The listing builds one solid part. Answer for the finished solid, in the listing's coordinates (mm). A direction names the side the tool comes from. Give positions to 0.01 mm unless a question says otherwise; leave off trailing zeros. Loops run counter-clockwise (first coordinate to the right, second up) from the corner with the lowest first, then second, coordinate; pieces in that order, holes last.
Item 1: A tool of negligible diameter and unlimited length cuts with its end or side. For faces 1 (the face through (5.7, 17, 0)), 2 (the face through (0, 1.1, 2.7)), from which of +Z, -Z, +X, -X, +Y, -Y can it reach the whole face along a straight path? Write none if from no direction.
Item 2: Consider line 1 along Z through (x, y) = (0, 1.5); line 2 along Y through (x, z) = (4, -4.5); line 3 along Y through (x, z) = (1.25, -2). Determine where each line is inside the solid, lowest interval first.
Item 3: Section C-C, the plane y = 11.25 is taken. Give the vertices of the cut face in (x, z).
Item 4: Section D-D, the plane z = 4.5 is taken. Give the vertices of the cut face in (x, y).
Item 5: The mould has two halves that part along Z. Classify faces 3 (the face through (-5.15, 11.5, -0.08)), 4 (the face through (0, 5, -1.7)), 5 (the face through (0, 17, -5.7)): pulls with the +Z half, pulls with the -Z half, needs draft (parallel to the pull), parting line crosses it, or undercut.
Item 6: Each of these flat-tipped pins is pushed along its axis until it touches: pin 1 Ø5 at (x, y) = (0.5, 4.5) entering from -Z; pin 2 Ø1.1 at (y, z) = (4, 0.5) entering from +X; pin 3 Ø1.1 at (y, z) = (2.5, 0.5) entering from -X. Where does it stop, or does it pass through?
Item 7: Section A-A, the plane y = 7.75 is taken. Give the vertices of the cut face in (x, z) (1 decimal).
Item 8: Section B-B, the plane x = 0 is taken. Give the vertices of the cut face in (y, z), and give its area (3 significant figures).
Autodesk Inventor part; units mm, degrees
ref_plane "YZ Plane" through (0, 0, 0) normal (1, 0, 0) x (0, 1, 0)
ref_plane "XZ Plane" through (0, 0, 0) normal (0, 1, 0) x (-1, 0, 0)
ref_plane "XY Plane" through (0, 0, 0) normal (0, 0, 1) x (1, 0, 0)
sketch "Sketch1" plane through (0, 0, 0) normal (0, 1, 0) x (-1, 0, 0)
  line L0 (14.5, -14.5) -> (-14.5, -14.5)
  line L1 (-14.5, -14.5) -> (-14.5, 14.5)
  line L2 (-14.5, 14.5) -> (14.5, 14.5)
  line L3 (14.5, 14.5) -> (14.5, -14.5)
  circle A0 centre (0, 0) radius 4
  dimension "d11" = 29
  dimension "d14" = 29
  dimension "d31" = 8
extrude "Extrusion1" add sketch "Sketch1" along normal blind 11.5 contours A0
sketch "Sketch2" plane through (0, 11.5, 0) normal (0, 1, 0) x (1, 0, 0)
  line L0 (-5.7, 5.7) -> (5.7, 5.7)
  line L1 (5.7, 5.7) -> (5.7, -5.7)
  line L2 (5.7, -5.7) -> (-5.7, -5.7)
  line L3 (-5.7, -5.7) -> (-5.7, 5.7)
  line L4 (14.5, 14.5) -> (-14.5, 14.5)
  line L5 (14.5, -14.5) -> (14.5, 14.5)
  line L6 (-14.5, -14.5) -> (14.5, -14.5)
  line L7 (-14.5, 14.5) -> (-14.5, -14.5)
  point P0 (0, 0)
  dimension "d15" = 8.8
  dimension "d16" = 8.8
  dimension "d17" = 8.8
  dimension "d18" = 8.8
  dimension "d32" = 11.4
extrude "Extrusion2" add sketch "Sketch2" along normal blind 11 contours L0 L1 L2 L3
sketch "Sketch3" plane through (0, 0, 0) normal (0, -1, 0) x (1, 0, 0)
  line L0 (-0.0005, -0.0003) -> (-0.0005, -1.7003)
  line L1 (-0.0005, -1.7003) -> (2.6995, -1.7003)
  line L2 (2.6995, -1.7003) -> (2.6995, 1.6997)
  line L3 (2.6995, 1.6997) -> (-2.7005, 1.6997)
  line L4 (-2.7005, 1.6997) -> (-2.7005, -1.7003)
  line L5 (-2.7005, -1.7003) -> (-0.0005, -1.7003)
  dimension "d42" = 1.7
  dimension "d43" = 2.7
  dimension "d44" = 3.4
  dimension "d45" = 5.4
extrude "Extrusion3" cut sketch "Sketch3" against normal blind 8.2
sketch "Sketch5" plane through (0, 0, 0) normal (0, -1, 0) x (1, 0, 0)
  circle A0 centre (0, 0) radius 2.7
  dimension "d35" = 5.4
extrude "Extrusion4" cut sketch "Sketch5" against normal blind 2.2
fillet "Fillet1" radius 0.635 4 edges at (2.6995, 4.1, 1.6997) (2.6995, 4.1, -1.7003) (-2.7005, 4.1, -1.7003) (-2.7005, 4.1, 1.6997)
sketch "Sketch6" plane through (0, 11.5, 0) normal (0, -1, 0) x (1, 0, 0)
  circle A0 centre (0, 0) radius 5
  dimension "d47" = 10
extrude "Extrusion5" add sketch "Sketch6" along normal up to surface (3.3 mm away)
equation "\"d14\" = d11"
equation "\"d16\" = d15"
equation "\"d17\" = d15"
equation "\"d18\" = d15"
equation "\"d42\" = 0.5 * d44"
properties part number "Motor_Key_Bearing_2_2"
Worked answers:
1. face 1: +Z, -Z, +X, +Y, -Y
1. face 2: -Y
2. line 1: z = -4 to -2.7, 2.7 to 4
2. line 2: y = 11.5 to 22.5
2. line 3: y = 2.2 to 22.5
3. outline: circle Ø10 at (0, 0)
4. outline: (-5.7, 11.5) - (-2.18, 11.5) - (-2.18, 8.2) - (2.18, 8.2) - (2.18, 11.5) - (5.7, 11.5) - (5.7, 22.5) - (-5.7, 22.5) - close
5. face 3: needs draft
5. face 4: undercut
5. face 5: pulls with the -Z half
6. pin 1: stops at z = -4
6. pin 2: stops at x = 4
6. pin 3: stops at x = -4
7. outline: circle Ø8 at (0, 0); hole (-2.7, -1.1) arc R0.6 ccw to (-2.1, -1.7) - (2.1, -1.7) arc R0.6 ccw to (2.7, -1.1) - (2.7, 1.1) arc R0.6 ccw to (2.1, 1.7) - (-2.1, 1.7) arc R0.6 ccw to (-2.7, 1.1) - close
8. outline: (0, -4) - (8.2, -4) - (8.2, -5) - (11.5, -5) - (11.5, -5.7) - (22.5, -5.7) - (22.5, 5.7) - (11.5, 5.7) - (11.5, 5) - (8.2, 5) - (8.2, 4) - (0, 4) - (0, 2.7) - (2.2, 2.7) - (2.2, 1.7) - (8.2, 1.7) - (8.2, -1.7) - (2.2, -1.7) - (2.2, -2.7) - (0, -2.7) - close
8. area: 192 mm2
